```python
from build123d import *

# Parameters (mm, degrees)
SKETCH_R        = 1
PAD_DEPTH       = 4
SKETCH001_W     = 101
SKETCH001_H     = 56
POCKET_DEPTH    = 2
SKETCH002_W     = 2
SKETCH002_H     = 65
POCKET001_DEPTH = 0.5


with BuildPart() as part:
    # Sketch → Pad (new body)
    with BuildSketch(Plane.XY):
        Polygon((105, 0), (105, 60), (82.5, 60), (82.5, 65), (77.5, 65), (77.5, 60), (27.5, 60), (27.5, 65), (22.5, 65), (22.5, 60), (0, 60), (0, 0), (22.5, 0), (22.5, -5), (27.5, -5), (27.5, 0), (77.5, 0), (77.5, -5), (82.5, -5), (82.5, 0), align=None)
        with Locations((25, 62.5)):
            Circle(SKETCH_R, mode=Mode.SUBTRACT)
        with Locations((80, 62.5)):
            Circle(SKETCH_R, mode=Mode.SUBTRACT)
        with Locations((80, -2.5)):
            Circle(SKETCH_R, mode=Mode.SUBTRACT)
        with Locations((25, -2.5)):
            Circle(SKETCH_R, mode=Mode.SUBTRACT)
    extrude(amount=PAD_DEPTH)

    # Sketch001 → Pocket (cut)
    with BuildSketch(Plane.XY):
        with Locations((52.5, 30)):
            Rectangle(SKETCH001_W, SKETCH001_H)
    extrude(amount=POCKET_DEPTH, mode=Mode.SUBTRACT)

    # Sketch002 (on Face5 of Pocket) → Pocket001 (cut)
    with BuildSketch(Plane.XY.offset(4)):
        with Locations((25, 30)):
            Rectangle(SKETCH002_W, SKETCH002_H)
        with Locations((80, 30)):
            Rectangle(SKETCH002_W, SKETCH002_H)
    extrude(amount=-POCKET001_DEPTH, mode=Mode.SUBTRACT)


solid = part.part
```
Here's how the part is built. I have some questions about the finished solid (model axes, mm). A direction names the side the tool comes from. Round coordinates to 2 decimals unless told otherwise and drop trailing zeros. Loops run counter-clockwise (first coordinate to the right, second up) from the corner with the lowest first, then second, coordinate; pieces in that order, holes last.
1. Thinking about a two-plate mould opening in Y: for faces 5 (the face through (11, 60, 2)), 6 (the face through (77.5, 63, 2)), 7 (the face through (25.46, -3.39, 1.97)), which applies, released by +Y, released by -Y, zero draft, split by the parting line, or undercut?
Answers:
face 5: released by +Y
face 6: zero draft
face 7: undercut
2. Suppose I cut it at A-A, the plane z = 1.3. Please give me the cut outline in (x, y), and give its area (3 significant figures).
Answers:
outline: (0, 0) - (22.5, 0) - (22.5, -5) - (27.5, -5) - (27.5, 0) - (77.5, 0) - (77.5, -5) - (82.5, -5) - (82.5, 0) - (105, 0) - (105, 60) - (82.5, 60) - (82.5, 65) - (77.5, 65) - (77.5, 60) - (27.5, 60) - (27.5, 65) - (22.5, 65) - (22.5, 60) - (0, 60) - close; hole (2, 2) - (103, 2) - (103, 58) - (2, 58) - close; hole circle Ø2 at (25, -2.5); hole circle Ø2 at (25, 62.5); hole circle Ø2 at (80, -2.5); hole circle Ø2 at (80, 62.5)
area: 731 mm2
3. Will these pins go through, and if not, where does the flat tip stop? pin 1 (1.2 mm diameter, centred on y = 62, z = 2, fed in from +X); pin 2 (5 mm diameter, centred on x = 55.5, y = 40, fed in from -Z); pin 3 (2 mm diameter, centred on y = 62, z = 2, fed in from -X).
Answers:
pin 1: stops at x = 82.5
pin 2: stops at z = 2
pin 3: stops at x = 22.5
4. For faces 1 (the face through (77.5, -2, 2)), 2 (the face through (11, 0, 2)), 3 (the face through (22.5, 63, 2)), 4 (the face through (52, 58, 1)), which set-ups out of +Z, -Z, +X, -X, +Y, -Y let a thin tool reach every point of the face, with its end or its side?
Answers:
face 1: +Z, -Z, -Y
face 2: +Z, -Z, -X, -Y
face 3: +Z, -Z, -X, +Y
face 4: -Z
5. Suppose I cut it at C-C, the plane x = 85. Please give me the cut outline in (y, z), and give its area (3 significant figures).
Answers:
outline: (0, 0) - (2, 0) - (2, 2) - (58, 2) - (58, 0) - (60, 0) - (60, 4) - (0, 4) - close
area: 128 mm2
6. If I drill on probe 1 along X at (y, z) = (62.5, 2.2); probe 2 along X at (y, z) = (47.5, 0.8); probe 3 along Y at (x, z) = (25, 2.25), over which ranges is the centre line in solid material (lowest first)?
Answers:
probe 1: x = 22.5 to 24, 26 to 27.5, 77.5 to 79, 81 to 82.5
probe 2: x = 0 to 2, 103 to 105
probe 3: y = -5 to -3.5, -1.5 to 61.5, 63.5 to 65
7. Suppose I cut it at B-B, the plane y = 48.5. Please give me the cut outline in (x, z).
Answers:
outline: (0, 0) - (2, 0) - (2, 2) - (103, 2) - (103, 0) - (105, 0) - (105, 4) - (81, 4) - (81, 3.5) - (79, 3.5) - (79, 4) - (26, 4) - (26, 3.5) - (24, 3.5) - (24, 4) - (0, 4) - close
